Check sheet for the modelled part. Datum: model origin and axes. Units: mm. A direction names the side the tool comes from. Give positions to 0.01 mm unless a question says otherwise; leave off trailing zeros. Write each loop counter-clockwise with the first axis right and the second up, starting at its lowest first coordinate (ties: lowest second). Pieces come first, ordered by that corner, then holes. Notation, with made-up numbers: (19, 14.5) -> (78, 14.5) arc R9 ccw to (78, 22.5) -> close; hole circle Ø1 at (7, 28.25). An arc over 180 degrees is marked (long way). Write each question's results on one line, items separated by ' | '. Start each with the question number.
```python
from build123d import *

# Parameters (mm, degrees)
F0_R     = 6.35
F1_DEPTH = 107.95
F2_DEPTH = 101.6


with BuildPart() as f1:
    # F0 (on Top) → F1 (new body)
    with BuildSketch(Plane.XY):
        Polygon((42.274462, 13.735805), (48.334151, 15.634893), (35.960805, 26.127054), (41.137061, 29.805741), (26.127054, 35.960805), (29.91319, 41.058995), (13.735805, 42.274462), (15.761207, 48.293109), (0, 44.45), (0, 50.758937), (-13.735805, 42.274462), (-15.634893, 48.334151), (-26.127054, 35.960805), (-29.805741, 41.137061), (-35.960805, 26.127054), (-41.058995, 29.91319), (-42.274462, 13.735805), (-48.293109, 15.761207), (-44.45, 0), (-50.799957, 0.066407), (-42.274462, -13.735805), (-48.334151, -15.634893), (-35.960805, -26.127054), (-41.137061, -29.805741), (-26.127054, -35.960805), (-29.91319, -41.058995), (-13.735805, -42.274462), (-15.761207, -48.293109), (0, -44.45), (0, -50.758937), (13.735805, -42.274462), (15.634893, -48.334151), (26.127054, -35.960805), (29.805741, -41.137061), (35.960805, -26.127054), (41.058995, -29.91319), (42.274462, -13.735805), (48.293109, -15.761207), (44.45, 0), (50.799957, -0.066407), align=None)
        Circle(F0_R, mode=Mode.SUBTRACT)
    extrude(amount=F1_DEPTH)

    # F0 (on Top) → F2 (join)
    with BuildSketch(Plane.XY):
        with BuildLine():
            ThreePointArc((50.799957, -0.066407), (50.799989, -0.033204), (50.8, 0))
            ThreePointArc((50.8, 0), (50.179751, 7.914074), (48.334151, 15.634893))
            Line((48.334151, 15.634893), (42.274462, 13.735805))
            Line((42.274462, 13.735805), (50.799957, -0.066407))
        make_face()
        with BuildLine():
            Line((35.960805, 26.127054), (48.334151, 15.634893))
            ThreePointArc((48.334151, 15.634893), (45.293241, 23.003528), (41.137061, 29.805741))
            Line((41.137061, 29.805741), (35.960805, 26.127054))
        make_face()
        with BuildLine():
            ThreePointArc((48.293109, -15.761207), (50.164136, -8.012454), (50.799957, -0.066407))
            Line((50.799957, -0.066407), (44.45, 0))
            Line((44.45, 0), (48.293109, -15.761207))
        make_face()
        with BuildLine():
            Line((26.127054, 35.960805), (41.137061, 29.805741))
            ThreePointArc((41.137061, 29.805741), (35.967951, 35.874037), (29.91319, 41.058995))
            Line((29.91319, 41.058995), (26.127054, 35.960805))
        make_face()
        with BuildLine():
            ThreePointArc((41.058995, -29.91319), (45.232944, -23.121867), (48.293109, -15.761207))
            Line((48.293109, -15.761207), (42.274462, -13.735805))
            Line((42.274462, -13.735805), (41.058995, -29.91319))
        make_face()
        with BuildLine():
            Line((13.735805, 42.274462), (29.91319, 41.058995))
            ThreePointArc((29.91319, 41.058995), (23.121867, 45.232944), (15.761207, 48.293109))
            Line((15.761207, 48.293109), (13.735805, 42.274462))
        make_face()
        with BuildLine():
            ThreePointArc((29.805741, -41.137061), (35.874037, -35.967951), (41.058995, -29.91319))
            Line((41.058995, -29.91319), (35.960805, -26.127054))
            Line((35.960805, -26.127054), (29.805741, -41.137061))
        make_face()
        with BuildLine():
            Line((0, 44.45), (15.761207, 48.293109))
            ThreePointArc((15.761207, 48.293109), (8.012454, 50.164136), (0.066407, 50.799957))
            Line((0.066407, 50.799957), (0, 50.758937))
            Line((0, 50.758937), (0, 44.45))
        make_face()
        with BuildLine():
            ThreePointArc((15.634893, -48.334151), (23.003528, -45.293241), (29.805741, -41.137061))
            Line((29.805741, -41.137061), (26.127054, -35.960805))
            Line((26.127054, -35.960805), (15.634893, -48.334151))
        make_face()
        with BuildLine():
            Line((0, 50.758937), (0.066407, 50.799957))
            ThreePointArc((0.066407, 50.799957), (0.033204, 50.799989), (0, 50.8))
            Line((0, 50.8), (0, 50.758937))
        make_face()
        with BuildLine():
            ThreePointArc((0, -50.8), (7.914074, -50.179751), (15.634893, -48.334151))
            Line((15.634893, -48.334151), (13.735805, -42.274462))
            Line((13.735805, -42.274462), (0, -50.758937))
            Line((0, -50.758937), (0, -50.8))
        make_face()
        with BuildLine():
            Line((0, 50.758937), (0, 50.8))
            ThreePointArc((0, 50.8), (-7.914074, 50.179751), (-15.634893, 48.334151))
            Line((-15.634893, 48.334151), (-13.735805, 42.274462))
            Line((-13.735805, 42.274462), (0, 50.758937))
        make_face()
        with BuildLine():
            ThreePointArc((-0.066407, -50.799957), (-0.033204, -50.799989), (0, -50.8))
            Line((0, -50.8), (0, -50.758937))
            Line((0, -50.758937), (-0.066407, -50.799957))
        make_face()
        with BuildLine():
            Line((-26.127054, 35.960805), (-15.634893, 48.334151))
            ThreePointArc((-15.634893, 48.334151), (-23.003528, 45.293241), (-29.805741, 41.137061))
            Line((-29.805741, 41.137061), (-26.127054, 35.960805))
        make_face()
        with BuildLine():
            ThreePointArc((-15.761207, -48.293109), (-8.012454, -50.164136), (-0.066407, -50.799957))
            Line((-0.066407, -50.799957), (0, -50.758937))
            Line((0, -50.758937), (0, -44.45))
            Line((0, -44.45), (-15.761207, -48.293109))
        make_face()
        with BuildLine():
            Line((-35.960805, 26.127054), (-29.805741, 41.137061))
            ThreePointArc((-29.805741, 41.137061), (-35.874037, 35.967951), (-41.058995, 29.91319))
            Line((-41.058995, 29.91319), (-35.960805, 26.127054))
        make_face()
        with BuildLine():
            ThreePointArc((-29.91319, -41.058995), (-23.121867, -45.232944), (-15.761207, -48.293109))
            Line((-15.761207, -48.293109), (-13.735805, -42.274462))
            Line((-13.735805, -42.274462), (-29.91319, -41.058995))
        make_face()
        with BuildLine():
            Line((-42.274462, 13.735805), (-41.058995, 29.91319))
            ThreePointArc((-41.058995, 29.91319), (-45.232944, 23.121867), (-48.293109, 15.761207))
            Line((-48.293109, 15.761207), (-42.274462, 13.735805))
        make_face()
        with BuildLine():
            ThreePointArc((-41.137061, -29.805741), (-35.967951, -35.874037), (-29.91319, -41.058995))
            Line((-29.91319, -41.058995), (-26.127054, -35.960805))
            Line((-26.127054, -35.960805), (-41.137061, -29.805741))
        make_face()
        with BuildLine():
            Line((-44.45, 0), (-48.293109, 15.761207))
            ThreePointArc((-48.293109, 15.761207), (-50.164136, 8.012454), (-50.799957, 0.066407))
            Line((-50.799957, 0.066407), (-44.45, 0))
        make_face()
        with BuildLine():
            ThreePointArc((-48.334151, -15.634893), (-45.293241, -23.003528), (-41.137061, -29.805741))
            Line((-41.137061, -29.805741), (-35.960805, -26.127054))
            Line((-35.960805, -26.127054), (-48.334151, -15.634893))
        make_face()
        with BuildLine():
            Line((-42.274462, -13.735805), (-50.799957, 0.066407))
            ThreePointArc((-50.799957, 0.066407), (-50.184913, -7.881274), (-48.334151, -15.634893))
            Line((-48.334151, -15.634893), (-42.274462, -13.735805))
        make_face()
    extrude(amount=F2_DEPTH)


solid = f1.part
```
Item 1: Mould release check, pull along Y, two halves, no side actions. Record for faces 5 (the flat face through (42.23, 20.81, 104.73)), 6 (the cylindrical face through (-45.182, 23.221, 50.089)), 7 (the cylindrical face through (-23.221, -45.182, 50.089)): pulls with the +Y half, pulls with the -Y half, needs draft (parallel to the pull), parting line crosses it, or undercut.
Item 2: Thickness scan on probe 1 along Z at (x, y) = (-39, -28); probe 2 along Y at (x, z) = (39, 52); probe 3 along Y at (x, z) = (8.5, 78.5). Record the ranges inside material, lowest first. Write a range as from..to.
Item 3: Section check A-A on z = 43.5. Record the boundary of the cut face in (x, y), then the cut area to 3 significant figures.
Item 4: Section check D-D on x = -20. Record the boundary of the cut face in (y, z), then the cut area to 3 significant figures.
Item 5: Section check C-C on x = -2. Record the boundary of the cut face in (y, z).
Item 6: Section check B-B on y = 3. Record the boundary of the cut face in (x, z).
Item 7: Set-up check for faces 1 (the flat face through (11, 1, 107.95)), 2 (the flat face through (-38.47, 27.99, 104.73)), 3 (the flat face through (-46.4, 8, 104.7)), 4 (the flat face through (3.2, -49.3, 101.6)): record each of +Z, -Z, +X, -X, +Y, -Y from which the full face is reachable in a straight line by a thin tool's end or side.
Item 8: Depth check by flat-ended pin: pin 1 Ø6 at (x, y) = (18.5, 45.5) entering from +Z; pin 2 Ø3 at (y, z) = (48.5, 104.5) entering from +X; pin 3 Ø12 at (x, z) = (-10.5, 42.5) entering from -Y; pin 4 Ø11.5 at (x, y) = (0, 0) entering from +Z. Enter the tip coordinate at first touch or a pass-through.
Check sheet entries:
1) face 5: undercut | face 6: pulls with the +Y half | face 7: pulls with the -Y half
2) probe 1: z = 0..101.6 | probe 2: y = -32.55..32.55 | probe 3: y = -50.08..50.08
3) outline: (-50.8, 0.07) arc R50.8 ccw to (-48.33, -15.63) arc R50.8 ccw to (-41.14, -29.81) arc R50.8 ccw to (-29.91, -41.06) arc R50.8 ccw to (-15.76, -48.29) arc R50.8 ccw to (-0.07, -50.8) arc R52.5 ccw to (0, -50.8) arc R50.8 ccw to (15.63, -48.33) arc R50.8 ccw to (29.81, -41.14) arc R50.8 ccw to (41.06, -29.91) arc R50.8 ccw to (48.29, -15.76) arc R50.8 ccw to (50.8, -0.07) arc R52.5 ccw to (50.8, 0) arc R50.8 ccw to (48.33, 15.63) arc R50.8 ccw to (41.14, 29.81) arc R50.8 ccw to (29.91, 41.06) arc R50.8 ccw to (15.76, 48.29) arc R50.8 ccw to (0.07, 50.8) arc R52.5 ccw to (0, 50.8) arc R50.8 ccw to (-15.63, 48.33) arc R50.8 ccw to (-29.81, 41.14) arc R50.8 ccw to (-41.06, 29.91) arc R50.8 ccw to (-48.29, 15.76) arc R50.8 ccw to start; hole circle Ø12.7 at (0, 0) | area: 7,980 mm^2
4) outline: (-46.7, 0) -> (46.7, 0) -> (46.7, 101.6) -> (43.19, 101.6) -> (43.19, 107.95) -> (-41.8, 107.95) -> (-41.8, 101.6) -> (-46.7, 101.6) -> close | area: 10,000 mm^2
5) outline: (-50.76, 0) -> (-6.03, 0) -> (-6.03, 107.95) -> (-44.94, 107.95) -> (-44.94, 101.6) -> (-50.76, 101.6) -> close; (6.03, 0) -> (50.76, 0) -> (50.76, 101.6) -> (49.52, 101.6) -> (49.52, 107.95) -> (6.03, 107.95) -> close
6) outline: (-50.71, 0) -> (-5.6, 0) -> (-5.6, 107.95) -> (-45.18, 107.95) -> (-45.18, 101.6) -> (-50.71, 101.6) -> close; (5.6, 0) -> (50.71, 0) -> (50.71, 101.6) -> (48.91, 101.6) -> (48.91, 107.95) -> (5.6, 107.95) -> close
7) face 1: +Z, +X, -X, +Y, -Y | face 2: +Z, +Y | face 3: +Z, -X | face 4: +Z, -Y
8) pin 1: stops at z = 101.6 | pin 2: stops at x = 15.76 | pin 3: stops at y = -50.6 | pin 4: passes through
